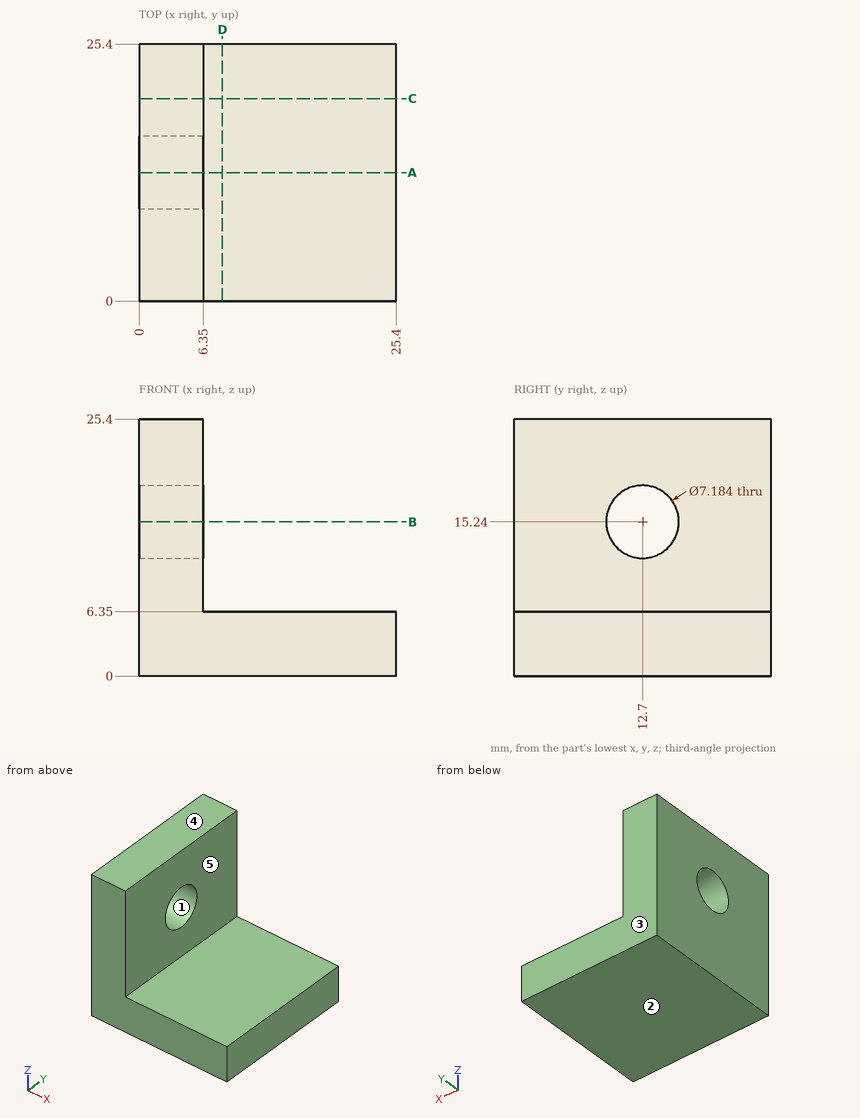
Geometry check sheet. Reference: drawing and pictorial views, mm from the part's lowest x, y, z. A direction names the side the tool comes from. Give positions to 0.01 mm unless a question says otherwise; leave off trailing zeros. Order: outer loops, then holes, each group sorted by start corner. A loop starts at its lowest first (then second) coordinate and runs counter-clockwise, first axis right, second up. Notation, with made-up numbers: M 78,45 L 90,45 A10 cw 90,49 Z; hole C -11.5,53 d5. An arc over 180 degrees is marked long. Answer in a Markdown table with one row per item. Add a question column.
Item 1: Section check C-C, the plane y = 20. Enter the section's corners in (x, z), and give its area (3 significant figures).
Item 2: Scan lines: probe 1 along Z at (x, y) = (4.5, 12.7); probe 2 along Z at (x, y) = (22.5, 20.25). Record each from-to range of solid material in increasing order. Write a range as from..to.
Item 3: Section check B-B, the plane z = 15.24. Enter the section's corners in (x, y).
Item 4: Mould release check, pull along Y, two halves, no side actions. Record for the marked faces 1, 2 and 3: released by +Y, released by -Y, zero draft, split by the parting line, or undercut.
Item 5: Gauge pin test, flat ends, axial feed: pin 1 (15 mm diameter, centred on x = 14, y = 18.5, fed in from +Z); pin 2 (4.5 mm diameter, centred on y = 12.7, z = 15.24, fed in from +X); pin 3 (10 mm diameter, centred on y = 9.5, z = 21, fed in from +X). Record the tip position at first contact, or that the pin passes through.
Item 6: Tool access check on the marked faces 4 and 5. Record the directions out of +Z, -Z, +X, -X, +Y, -Y that give a thin tool (end or side, any length) a straight path to the whole face; none if there is none.
Item 7: Section check A-A, the plane y = 12.7. Enter the section's corners in (x, z).
Item 8: Section check D-D, the plane x = 8.25. Enter the section's corners in (y, z), and give its area (3 significant figures).
Filled sheet:
| question | item | result |
|---|---|---|
| 1 | outline | M 0,0 L 25.4,0 L 25.4,6.35 L 6.35,6.35 L 6.35,25.4 L 0,25.4 Z |
| 1 | area | 282 mm^2 |
| 2 | probe 1 | z = 0..11.65, 18.83..25.4 |
| 2 | probe 2 | z = 0..6.35 |
| 3 | outline | M 0,0 L 6.35,0 L 6.35,9.11 L 0,9.11 Z; M 0,16.29 L 6.35,16.29 L 6.35,25.4 L 0,25.4 Z |
| 4 | face 1 | undercut |
| 4 | face 2 | zero draft |
| 4 | face 3 | released by +Y |
| 5 | pin 1 | stops at z = 6.35 |
| 5 | pin 2 | passes through |
| 5 | pin 3 | stops at x = 6.35 |
| 6 | face 4 | +Z, +X, -X, +Y, -Y |
| 6 | face 5 | +Z, +X, +Y, -Y |
| 7 | outline | M 0,0 L 25.4,0 L 25.4,6.35 L 6.35,6.35 L 6.35,11.65 L 0,11.65 Z; M 0,18.83 L 6.35,18.83 L 6.35,25.4 L 0,25.4 Z |
| 8 | outline | M 0,0 L 25.4,0 L 25.4,6.35 L 0,6.35 Z |
| 8 | area | 161 mm^2 |
